```python
from build123d import *

# Parameters (mm, degrees)
BOSS_EXTRUDE1_DEPTH = 20
CUT_EXTRUDE1_DEPTH  = 7.5
FILLET1_R           = 30
FILLET2_R           = 1
FILLET3_R           = 2
SKETCH6_R           = 1
CUT_EXTRUDE2_DEPTH  = 15


with BuildPart() as part:
    # Sketch1 → Boss-Extrude1 (new body)
    with BuildSketch(Plane(origin=(0, 0, 0), x_dir=(1, 0, 0), z_dir=(0, 1, 0))):
        with BuildLine():
            Line((-100, 32.5), (100, 32.5))
            ThreePointArc((100, 32.5), (132.5, 0), (100, -32.5))
            Line((100, -32.5), (-100, -32.5))
            ThreePointArc((-100, -32.5), (-132.5, 0), (-100, 32.5))
        make_face()
    extrude(amount=BOSS_EXTRUDE1_DEPTH)

    # Sketch2 → Cut-Extrude1 (cut)
    with BuildSketch(Plane(origin=(0, 20, 0), x_dir=(1, 0, 0), z_dir=(0, 1, 0))):
        with BuildLine():
            Line((-100, -30.5), (100, -30.5))
            ThreePointArc((100, -30.5), (130.5, 0), (100, 30.5))
            Line((100, 30.5), (-100, 30.5))
            ThreePointArc((-100, 30.5), (-130.5, 0), (-100, -30.5))
        make_face()
    extrude(amount=-CUT_EXTRUDE1_DEPTH, mode=Mode.SUBTRACT)

    # Fillet1
    # the kernel refuses this fillet: 30 mm, written as the material it adds along each edge
    with BuildSketch(Plane(origin=(100, 12.5, -30.5), x_dir=(0, 1, 0), z_dir=(-1, 0, 0)), Plane(origin=(-100, 12.5, 30.5), x_dir=(0, 1, 0), z_dir=(1, 0, 0))) as fillet1_piece_1:
        with BuildLine():
            CenterArc((30, -19.843134833), FILLET1_R, 138.590377891, 41.409622109)
            Line((0, -19.843134833), (-0.6, -19.843134833))
            Line((-0.6, -19.843134833), (-0.6, 0))
            Line((-0.6, 0), (0, 0.6))
            ThreePointArc((0, 0.6), (3.75, 0.6), (7.05, 0.396862697))
            Line((7.05, 0.396862697), (7.5, 0))
        make_face()
    extrude(amount=200)
    with BuildSketch(Plane(origin=(-100, 12.5, 0), x_dir=(0, 0, -1), z_dir=(1, 0, 0))) as fillet1_piece_2:
        with BuildLine():
            CenterArc((10.656865167, 30), FILLET1_R, 270, 41.409622109)
            Line((10.656865167, 0), (10.656865167, -0.6))
            Line((10.656865167, -0.6), (30.5, -0.6))
            Line((30.5, -0.6), (31.1, 0))
            ThreePointArc((31.1, 0), (31.1, 3.75), (30.896862697, 7.05))
            Line((30.896862697, 7.05), (30.5, 7.5))
        make_face()
    revolve(axis=Axis((-100, 12.5, 0), (0, 1, 0)), revolution_arc=180)
    with BuildSketch(Plane(origin=(100, 12.5, 0), x_dir=(0, 0, 1), z_dir=(-1, 0, 0))) as fillet1_piece_3:
        with BuildLine():
            CenterArc((10.656865167, 30), FILLET1_R, 270, 41.409622109)
            Line((10.656865167, 0), (10.656865167, -0.6))
            Line((10.656865167, -0.6), (30.5, -0.6))
            Line((30.5, -0.6), (31.1, 0))
            ThreePointArc((31.1, 0), (31.1, 3.75), (30.896862697, 7.05))
            Line((30.896862697, 7.05), (30.5, 7.5))
        make_face()
    revolve(axis=Axis((100, 12.5, 0), (0, 1, 0)), revolution_arc=180)

    # Fillet2
    fillet2_edges = [part.edges().sort_by_distance(p)[0] for p in [
        (132.5, 20, 0),
        (0, 20, -32.5),
        (-130.5, 20, 0),
        (0, 20, 30.5),
        (130.5, 20, 0),
        (0, 20, -30.5),
        (-132.5, 20, 0),
        (0, 20, 32.5),
    ]]
    fillet(fillet2_edges, radius=FILLET2_R)

    # Fillet3
    fillet3_edges = [part.edges().sort_by_distance(p)[0] for p in [
        (0, 0, -32.5),
        (132.5, 0, 0),
        (0, 0, 32.5),
        (-132.5, 0, 0),
    ]]
    fillet(fillet3_edges, radius=FILLET3_R)

    # Sketch4 → Revolve1 (revolve)
    with BuildSketch(Plane.XY):
        with BuildLine():
            Line((-100, 12), (-100, 42))
            ThreePointArc((-100, 42), (-115, 27), (-100, 12))
        make_face()
    revolve(axis=Axis((-100, 12, 0), (0, 1, 0)))

    # Sketch6 → Cut-Extrude2 (cut)
    with BuildSketch(Plane(origin=(-25.893398282, -25.893398282, 0), x_dir=(0.7071067811865488, -0.7071067811865464, 0), z_dir=(0.7071067811865464, 0.7071067811865488, 0))):
        with Locations(Location((-89.802561211, 0, 0), (0, 0, 180))):
            Circle(SKETCH6_R)
    extrude(amount=-CUT_EXTRUDE2_DEPTH, mode=Mode.SUBTRACT)


solid = part.part
```
Check sheet for the modelled part. Datum: model origin and axes. Units: mm. Give positions to 0.01 mm unless a question says otherwise; leave off trailing zeros. Write each loop counter-clockwise with the first axis right and the second up, starting at its lowest first coordinate (ties: lowest second). Pieces come first, ordered by that corner, then holes.
Item 1: Cross-section at B-B (y = 9). Enter the section's corners in (x, z).
Item 2: Gauge pin test, flat ends, axial feed: pin 1 (10 mm diameter, centred on y = 6, z = 1, fed in from +X); pin 2 (2 mm diameter, centred on y = 12.5, z = 18, fed in from -X); pin 3 (3 mm diameter, centred on x = 51, z = 18.5, fed in from +Y). Record the tip position at first contact, or that the pin passes through.
Item 3: Cross-section at A-A (x = 96.5). Enter the section's corners in (y, z).
Item 4: Scan lines: L1, parallel to X at y = 18, z = 0.5; L2, parallel to Z at x = 19, y = 19; L3, parallel to Y at x = -2, z = -6.5. Record each from-to range of solid material in increasing order.
Item 5: Cross-section at C-C (x = -95). Count the separate pieces of the cut face and the enclosed holes in it, and give its area (3 significant figures).
Item 6: Draft check along Y on faces 1 (the face through (132.492, 10.381, -0.715)), 2 (the face through (-95.31, 33.04, 0.3)), 3 (the face through (2, 0, 0)). Enter one of: released by +Y, released by -Y, zero draft, split by the parting line, or undercut.
Report:
1. outline: (-100, -32.5) - (100, -32.5) arc R32.5 ccw to (100, 32.5) - (-100, 32.5) arc R32.5 ccw to start
2. pin 1: stops at x = 132.5
2. pin 2: stops at x = -127.7
2. pin 3: stops at y = 13.99
3. outline: (0, -30.5) arc R2 ccw to (2, -32.5) - (19, -32.5) arc R1 ccw to (20, -31.5) - (20, -30.87) arc R1 ccw to (19.76, -30.22) arc R30 cw to (12.5, -10.66) - (12.5, 10.66) arc R30 cw to (19.76, 30.22) arc R1 ccw to (20, 30.87) - (20, 31.5) arc R1 ccw to (19, 32.5) - (2, 32.5) arc R2 ccw to (0, 30.5) - close
4. L1: x = -132.5 to -127.97, -111.99 to -88.01, 127.97 to 132.5
4. L2: z = -32.5 to -29.3, 29.3 to 32.5
4. L3: y = 0 to 12.5
5. separate pieces: 2
5. enclosed holes: 1
5. area: 1,560 mm2
6. face 1: zero draft
6. face 2: undercut
6. face 3: released by -Y
